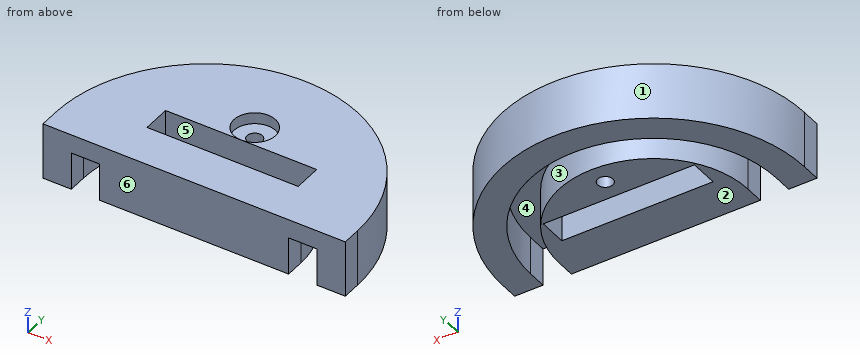
Autodesk Inventor part; units mm, degrees
ref_plane "YZ Plane" through (0, 0, 0) normal (1, 0, 0) x (0, 1, 0)
ref_plane "XZ Plane" through (0, 0, 0) normal (0, 1, 0) x (-1, 0, 0)
ref_plane "XY Plane" through (0, 0, 0) normal (0, 0, 1) x (1, 0, 0)
sketch "Sketch2" plane through (0, 0, 0) normal (0, 0, 1) x (1, 0, 0)
  arc A0 (31.75, 0) -> (-31.75, 0) centre (0, 0) ccw
  arc A1 (41.275, 0) -> (-41.275, 0) centre (0, 0) ccw
  line L0 (-41.275, 0) -> (-31.75, 0)
  line L1 (31.75, 0) -> (41.275, 0)
  arc A2 (50.8, 0) -> (-50.8, 0) centre (0, 0) ccw
  line L2 (-50.8, 0) -> (-41.275, 0)
  line L3 (41.275, 0) -> (50.8, 0)
  line L4 (-31.75, 0) -> (31.75, 0)
  line L5 (0, 0) -> (0, 31.75) construction
  line L6 (0, 8.255) -> (25.4, 8.255)
  line L7 (25.4, 8.255) -> (25.4, 17.78)
  line L8 (25.4, 17.78) -> (0, 17.78)
  line L9 (0, 17.78) -> (-25.4, 17.78)
  line L10 (-25.4, 17.78) -> (-25.4, 8.255)
  line L11 (-25.4, 8.255) -> (0, 8.255)
  dimension "d2" = 63.5
  dimension "d3" = 9.525
  dimension "d4" = 9.525
  dimension "d5" = 25.4
  dimension "d6" = 8.255
  dimension "d7" = 9.525
extrude "Extrusion1" add sketch "Sketch2" along normal blind 6.35
extrude "Extrusion2" add sketch "Sketch2" against normal blind 12.7 contours L4 A0 | A1 L2 A2 L3
sketch "Sketch5" plane through (0, 0, 6.35) normal (0, 0, 1) x (1, 0, 0)
  line L0 (-25.4, 17.78) -> (25.4, 17.78)
  arc A0 (31.75, 0) -> (-31.75, 0) centre (0, 0) ccw
  line L1 (0, 17.78) -> (0, 31.75) construction
  arc A1 (31.75, 0) -> (-31.75, 0) centre (0, 0) ccw construction
  point P0 (0, 24.765)
hole "Hole2" at (0, 24.765, 6.35) direction (0, 0, -1) diameter 5.1054 end through all counterbore diameter 13.97 counterbore depth 3.81
sketch "Sketch6" plane through (-50.8, 0, 6.35) normal (0, -1, 0) x (1, 0, 0)
  line L0 (101.6, 0) -> (101.6, -19.05)
  line L1 (0, -19.05) -> (0, 0)
  line L2 (101.6, 0) -> (0, 0)
  line L3 (0, 0) -> (0, -19.05)
  line L4 (9.525, -19.05) -> (0, -19.05)
  line L5 (0, -19.05) -> (9.525, -19.05)
  line L6 (9.525, -6.35) -> (19.05, -6.35)
  line L7 (9.525, -19.05) -> (9.525, -6.35)
  line L8 (19.05, -6.35) -> (19.05, -19.05)
  line L9 (9.525, -6.35) -> (19.05, -6.35)
  line L10 (19.05, -6.35) -> (19.05, -19.05)
  line L11 (19.05, -19.05) -> (82.1864, -19.05)
  line L12 (92.075, -19.05) -> (9.525, -19.05)
  line L13 (82.55, -6.35) -> (82.55, -19.05)
  line L14 (82.55, -6.35) -> (92.075, -6.35)
  line L15 (92.075, -6.35) -> (92.075, -19.05)
  line L16 (92.075, -6.35) -> (92.075, -19.05)
  line L17 (101.6, -19.05) -> (92.075, -19.05)
  line L18 (92.075, -19.05) -> (101.6, -19.05)
  line L19 (101.6, -19.05) -> (101.6, 0)
  point P0 (50.8, -6.35)
extrude "Extrusion3" add sketch "Sketch6" along normal blind 6.35 contours L0 L17 L15 L14 L13 L12 L11 L8 L6 L7 L4 L1 L2
equation "\"d2\" = insideDiameterOfRing"
equation "\"d3\" = innerRingWidth"
equation "\"d4\" = outerRingWidth"
equation "\"d5\" = halfWidthForPryBar"
equation "\"d7\" = depthForPryBar"
equation "\"d8\" = topPartHeight"
equation "\"d10\" = lowerPartHeight"
equation "\"insideDiameterOfRing\" = 63.5"
equation "\"wallThicknessOfRing\" = 9.525"
equation "\"outsideDiameterOfRing\" = insideDiameterOfRing + 2 * wallThicknessOfRing"
equation "\"widthForPryBar\" = 50.8"
equation "\"outerRingWidth\" = 9.525"
equation "\"innerRingWidth\" = 9.525"
equation "\"halfWidthForPryBar\" = 0.5 * widthForPryBar"
equation "\"distanceFromEdgeToPryBar\" = 8.255"
equation "\"totalHeightOfPart\" = 19.05"
equation "\"topPartHeight\" = 6.35"
equation "\"lowerPartHeight\" = totalHeightOfPart - topPartHeight"
equation "\"depthForPryBar\" = 9.525"
properties part number "dRingHolder" material "PBT Plastic"
Verification items for the finished model (mm, model axes). Face numbers are marked on the shaded views. A direction names the side the tool comes from. Coordinates: 2 decimals unless noted, no trailing zeros. Order: outer loops, then holes, each group sorted by start corner. A loop starts at its lowest first (then second) coordinate and runs counter-clockwise, first axis right, second up. Notation, with made-up numbers: (4, -22) -> (57, -22) arc R24 ccw to (57, 12) -> close; hole circle Ø7 at (42, 51). An arc over 180 degrees is marked (long way). Put each result on its own line as item: value. Start each with the question number.
1. Cross-section at A-A, the plane z = -5.5. Record the boundary of the cut face in (x, y) (3 decimals).
2. Access from +Z, -Z, +X, -X, +Y, -Y to the whole of each face (thin tool, end or side, straight path). Record for the marked faces 4, 5 and 6.
3. Cross-section at C-C, the plane y = 15. Record the boundary of the cut face in (x, z).
4. Cross-section at D-D, the plane x = -21.5. Record the boundary of the cut face in (y, z) (3 decimals), then the cut area to 3 significant figures.
5. Mould release check, pull along X, two halves, no side actions. Record for the marked faces 1, 2 and 3: released by +X, released by -X, zero draft, split by the parting line, or undercut.
6. Go/stop test with flat-tipped pins: pin 1 Ø15.5 at (x, y) = (0, 28) entering from +Z; pin 2 Ø1 at (y, z) = (43, -2) entering from -X; pin 3 Ø6 at (y, z) = (27.5, -4.5) entering from +X; pin 4 Ø1 at (y, z) = (15, -6.5) entering from -X. Record where each tip stops, or that it passes through.
7. Material ranges on L1, parallel to Y at x = 0, z = -8 (3 decimals); L2, parallel to X at y = 14, z = -11.75; L3, parallel to X at y = 15.5, z = -10, recorded low to high. Write a range as [from, to].
8. Cross-section at B-B, the plane x = -5. Record the boundary of the cut face in (y, z) (3 decimals).
Computed:
1. outline: (-50.8, -6.35) -> (-41.275, -6.35) -> (-41.275, 0) arc R41.275 cw to (41.275, 0) -> (41.275, -6.35) -> (50.8, -6.35) -> (50.8, 0) arc R50.8 ccw to (-50.8, 0) -> close; (-31.75, -6.35) -> (31.75, -6.35) -> (31.75, 0) arc R31.75 ccw to (-31.75, 0) -> close; hole (-25.4, 8.255) -> (25.4, 8.255) -> (25.4, 17.78) -> (-25.4, 17.78) -> close; hole circle Ø5.105 at (0, 24.765)
2. face 4: -Z
2. face 5: +Z, -Z
2. face 6: +Z, -Z, +X, -X, -Y
3. outline: (-48.53, -12.7) -> (-38.45, -12.7) -> (-38.45, 0) -> (-27.98, 0) -> (-27.98, -12.7) -> (-25.4, -12.7) -> (-25.4, 6.35) -> (-48.53, 6.35) -> close; (25.4, -12.7) -> (27.98, -12.7) -> (27.98, 0) -> (38.45, 0) -> (38.45, -12.7) -> (48.53, -12.7) -> (48.53, 6.35) -> (25.4, 6.35) -> close
4. outline: (-6.35, -12.7) -> (8.255, -12.7) -> (8.255, 6.35) -> (-6.35, 6.35) -> close; (17.78, -12.7) -> (23.363, -12.7) -> (23.363, 0) -> (35.233, 0) -> (35.233, -12.7) -> (46.026, -12.7) -> (46.026, 6.35) -> (17.78, 6.35) -> close
4. area: 666 mm2
5. face 1: split by the parting line
5. face 2: zero draft
5. face 3: undercut
6. pin 1: z = 6.35
6. pin 2: x = -27.83
6. pin 3: x = 44.5
6. pin 4: x = -48.69
7. L1: [-6.35, 8.255], [17.78, 22.212], [27.318, 31.75], [41.275, 50.8]
7. L2: [-48.83, -38.83], [-28.5, -25.4], [25.4, 28.5], [38.83, 48.83]
7. L3: [-48.38, -38.25], [-27.71, -25.4], [25.4, 27.71], [38.25, 48.38]
8. outline: (-6.35, -12.7) -> (8.255, -12.7) -> (8.255, 6.35) -> (-6.35, 6.35) -> close; (17.78, -12.7) -> (31.354, -12.7) -> (31.354, 0) -> (40.971, 0) -> (40.971, -12.7) -> (50.553, -12.7) -> (50.553, 6.35) -> (29.643, 6.35) -> (29.643, 2.54) -> (19.887, 2.54) -> (19.887, 6.35) -> (17.78, 6.35) -> close
